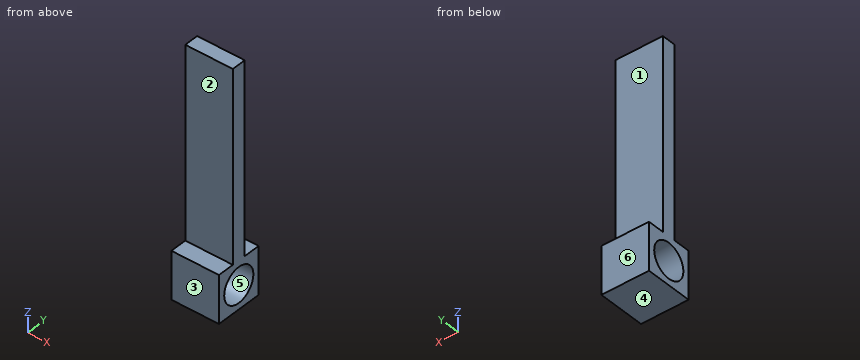
Autodesk Inventor part; units mm, degrees
ref_plane "YZ Plane" through (0, 0, 0) normal (1, 0, 0) x (0, 1, 0)
ref_plane "XZ Plane" through (0, 0, 0) normal (0, 1, 0) x (-1, 0, 0)
ref_plane "XY Plane" through (0, 0, 0) normal (0, 0, 1) x (1, 0, 0)
sketch "Sketch1" plane through (0, 0, 0) normal (0, 0, 1) x (1, 0, 0)
  line L0 (0, 0) -> (6.35, 0)
  line L1 (6.35, 0) -> (6.35, 1.905)
  line L2 (6.35, 1.905) -> (0, 1.905)
  line L3 (0, 1.905) -> (0, 0)
  dimension "d0" = 1.905
  dimension "d1" = 6.35
extrude "Extrusion1" add sketch "Sketch1" along normal blind 31.75
sketch "Sketch2" plane through (0, 1.905, 0) normal (0, 1, 0) x (1, 0, 0)
  line L0 (6.35, 0) -> (6.35, -31.75)
  line L1 (0, 0) -> (6.35, 0)
  line L2 (6.35, 0) -> (6.35, -6.35)
  line L3 (6.35, -6.35) -> (0, -6.35)
  line L4 (0, -6.35) -> (0, 0)
  dimension "d4" = 6.35
extrude "Extrusion2" add sketch "Sketch2" along normal blind 2.2225 and the other way blind 4.1275
sketch "Sketch3" plane through (6.35, 0, 31.75) normal (1, 0, 0) x (0, 0, -1)
  line L0 (21.2753, 0.9525) -> (48.2824, 0.9525) construction
  line L1 (28.575, 14.3554) -> (28.575, -13.5982) construction
  line L2 (31.75, 4.1275) -> (31.75, -2.2225) construction
  line L3 (25.4, 4.1275) -> (31.75, 4.1275) construction
  line L4 (31.75, -2.2225) -> (25.4, -2.2225) construction
  circle A0 centre (28.575, 0.9525) radius 2.3343
  point P0 (31.75, 0)
  dimension "d9" = 3.175
  dimension "d11" = 3.175
  dimension "d12" = 4.6685
extrude "Extrusion3" cut sketch "Sketch3" against normal through all
properties part number "000207"
The listing builds one solid part. Answer for the finished solid, in the listing's coordinates (mm). Face numbers are marked on the shaded views. A direction names the side the tool comes from. Give positions to 0.01 mm unless a question says otherwise; leave off trailing zeros. Write each loop counter-clockwise with the first axis right and the second up, starting at its lowest first coordinate (ties: lowest second). Pieces come first, ordered by that corner, then holes. Notation, with made-up numbers: (54.25, 77) - (66.25, 77) arc R33 cw to (66.25, 110) - close; hole circle Ø4 at (-27.5, 2.25). An arc over 180 degrees is marked (long way). Use one line per item in the form item = value. Start each with the question number.
1) The mould has two halves that part along Z. Classify the marked faces 4, 5 and 6: pulls with the +Z half, pulls with the -Z half, needs draft (parallel to the pull), parting line crosses it, or undercut.
2) Consider line 1 along Y through (x, z) = (4.75, 11) (3 decimals); line 2 along Z through (x, y) = (1, 3.5); line 3 along Y through (x, z) = (3.5, 3.5). Determine where each line is inside the solid, lowest interval first. Write a range as from..to.
3) Flat-ended cylindrical pins translate along their axes: pin 1 Ø1 at (x, z) = (3.5, 21.5) entering from +Y (3 decimals); pin 2 Ø1.5 at (x, z) = (4, 12.5) entering from -Y; pin 3 Ø0.7 at (x, y) = (4, -1) entering from +Z. Find the tip coordinate at first contact, or state that the pin passes through.
4) A tool of negligible diameter and unlimited length cuts with its end or side. For the marked faces 1, 2 and 3, from which of +Z, -Z, +X, -X, +Y, -Y can it reach the whole face along a straight path? Write none if from no direction.
5) Find section D-D on y = 3.75. Determine the outline of the cut face in (x, z).
6) Find section B-B on z = 2.5. Determine the outline of the cut face in (x, y).
7) Find section A-A on y = 0.5. Determine the outline of the cut face in (x, z).
Geometry results:
q1.face_4 = pulls with the -Z half
q1.face_5 = undercut
q1.face_6 = needs draft
q2.line_1 = 0..1.905
q2.line_2 = 0..6.35
q2.line_3 = -2.22..-1.36, 3.26..4.13
q3.pin_1 = 1.905
q3.pin_2 = 0
q3.pin_3 = 6.35
q4.face_1 = +Z, +X, -X, +Y
q4.face_2 = +Z, +X, -X, -Y
q4.face_3 = +Z, -Z, +X, -X, -Y
q5.outline = (0, 0) - (6.35, 0) - (6.35, 6.35) - (0, 6.35) - close
q6.outline = (0, -2.22) - (6.35, -2.22) - (6.35, -1.28) - (0, -1.28) - close; (0, 3.19) - (6.35, 3.19) - (6.35, 4.13) - (0, 4.13) - close
q7.outline = (0, 0) - (6.35, 0) - (6.35, 0.88) - (0, 0.88) - close; (0, 5.47) - (6.35, 5.47) - (6.35, 31.75) - (0, 31.75) - close
